from build123d import *

# Parameters (mm, degrees)
SKETCH005_R   = 1.15
PAD004_DEPTH  = 0.5
SKETCH006_R   = 1.775
SKETCH006_R_2 = 1.15
PAD005_DEPTH  = 1.75
FILLET002_R   = 0.1


with BuildPart() as part:
    # Sketch005 → Pad004 (new body)
    with BuildSketch(Plane.XZ):
        with BuildLine():
            Line((1.775, 0), (1.775, -4.225))
            Line((1.775, -4.225), (0.5, -3.925))
            Line((0.5, -3.925), (0.5, -7.925))
            Line((0.5, -7.925), (-0.5, -7.925))
            Line((-0.5, -7.925), (-0.5, -3.925))
            Line((-0.5, -3.925), (-1.775, -4.225))
            Line((-1.775, -4.225), (-1.775, 0))
            ThreePointArc((1.775, 0), (0, 1.775), (-1.775, 0))
        make_face()
        Circle(SKETCH005_R, mode=Mode.SUBTRACT)
    extrude(amount=PAD004_DEPTH)

    # Sketch006 (on Face11 of Pad004) → Pad005 (join)
    with BuildSketch(Plane.XZ.offset(0.5)):
        Circle(SKETCH006_R)
        Circle(SKETCH006_R_2, mode=Mode.SUBTRACT)
    extrude(amount=PAD005_DEPTH)

    # Fillet002
    fillet002_edges = [part.edges().sort_by_distance(p)[0] for p in [
        (-1.775, -2.25, 0),
        (-1.15, -2.25, 0),
    ]]
    fillet(fillet002_edges, radius=FILLET002_R)


with BuildPart() as part_1:
    # Body003 placement: moved
    add(part.part.moved(Location((0, 0.5, -8))))


solid = part_1.part
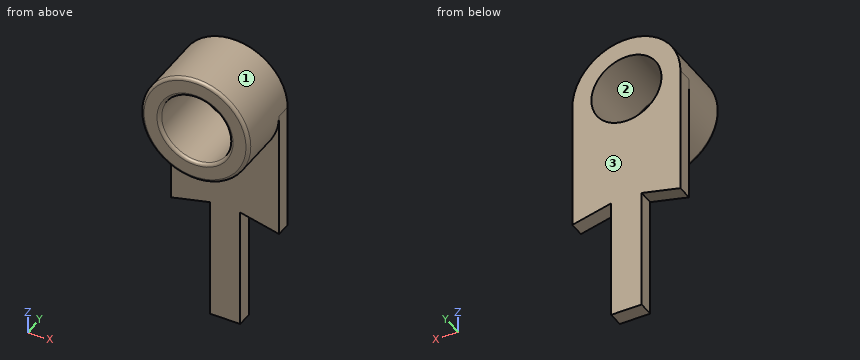
Input: part model. Units: mm. Frame: model coordinates. Face numbers are marked on the shaded views. Give positions to 0.01 mm unless a question says otherwise; leave off trailing zeros. Order: outer loops, then holes, each group sorted by start corner. A loop starts at its lowest first (then second) coordinate and runs counter-clockwise, first axis right, second up. Notation, with made-up numbers: (33, 28) - (71, 28) arc R25 cw to (71, 47) - close; hole circle Ø11 at (0.5, -37). An arc over 180 degrees is marked (long way). Answer as a JSON object with one key per item and string values. Group by question number.
Q1. Mould query, pull axis Z, two halves, no side actions, for the marked faces 1, 2 and 3. Classes: pulls with the +Z half, pulls with the -Z half, needs draft (parallel to the pull), parting line crosses it, or undercut.
Q2. Cut plane D-D, the plane z = -15.25. Output: boundary loops of the cut face in (x, y), then the cut area to 3 significant figures.
Q3. Cut plane B-B, the plane y = -1.3. Output: boundary loops of the cut face in (x, z) (3 decimals).
Q4. Cut plane A-A, the plane x = 0. Output: boundary loops of the cut face in (y, z) (3 decimals).
Q5. Line query: probe 1 along Z at (x, y) = (0, -0.9) (3 decimals); probe 2 along Y at (x, z) = (1, -12); probe 3 along Z at (x, y) = (-0.4, 0.3) (3 decimals). Output: solid intervals per line, ascending.
Q6. Cut plane C-C, the plane z = -11.25. Output: boundary loops of the cut face in (x, y) (3 decimals), then the cut area to 4 significant figures.
Results:
{
 "1": {"face 1": "parting line crosses it", "face 2": "undercut", "face 3": "needs draft"},
 "2": {"outline": "(-0.5, 0) - (0.5, 0) - (0.5, 0.5) - (-0.5, 0.5) - close", "area": "0.500 mm^2"},
 "3": {"outline": "circle Ø3.55 at (0, -8); hole circle Ø2.3 at (0, -8)"},
 "4": {"outline": "(-1.75, -9.675) arc R0.1 ccw to (-1.65, -9.775) - (0, -9.775) - (0, -15.925) - (0.5, -15.925) - (0.5, -9.15) - (-1.65, -9.15) arc R0.1 ccw to (-1.75, -9.25) - close; (-1.75, -6.75) arc R0.1 ccw to (-1.65, -6.85) - (0.5, -6.85) - (0.5, -6.225) - (-1.65, -6.225) arc R0.1 ccw to (-1.75, -6.325) - close"},
 "5": {"probe 1": "-9.775 to -9.15, -6.85 to -6.225", "probe 2": "0 to 0.5", "probe 3": "-15.925 to -9.078, -6.922 to -6.271"},
 "6": {"outline": "(-1.775, 0) - (1.775, 0) - (1.775, 0.5) - (-1.775, 0.5) - close", "area": "1.775 mm^2"}
}
